The model under review builds one solid part; all positions refer to its coordinate system, in mm. Give positions to 0.01 mm unless a question says otherwise; leave off trailing zeros. Loops run counter-clockwise (first coordinate to the right, second up) from the corner with the lowest first, then second, coordinate; pieces in that order, holes last. Notation, with made-up numbers: (50.5, 50.25) - (84.5, 50.25) arc R31 ccw to (84.5, 76.25) - close; hole circle Ø5 at (33, 48.25). An arc over 180 degrees is marked (long way). Return JSON: item names as keys, results as strings. Group by question number.
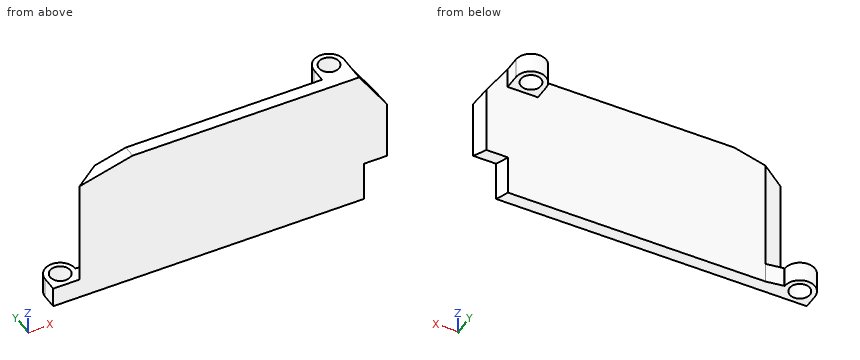
from build123d import *

# Parameters (mm, degrees)
EXTRUDE_1_DEPTH     = 14
CUT_EXTRUDE_1_DEPTH = 4
CUT_EXTRUDE_2_DEPTH = 23.370796565
EXTRUDE_2_DEPTH     = 2
EXTRUDE_3_DEPTH     = 2
MM_1_D              = 2
MM_2_D              = 2


with BuildPart() as part:
    # 草图2 → 凸台-拉伸1 (new body)
    with BuildSketch(Plane(origin=(0, 0, -2), x_dir=(-1, 0, 0), z_dir=(0, 0, -1))):
        with BuildLine():
            Line((-14.855557574, 24.75), (15.584929867, 24.75))
            Line((15.584929867, 24.75), (13.419866357, 26))
            Line((13.419866357, 26), (-14.208438024, 26))
            ThreePointArc((-14.208438024, 26), (-14.507523283, 25.36232965), (-14.855557574, 24.75))
        make_face()
    extrude(amount=EXTRUDE_1_DEPTH)

    # 草图3 → 切除-拉伸1 (cut)
    with BuildSketch(Plane(origin=(0, 0, -16), x_dir=(-1, 0, 0), z_dir=(0, 0, -1))):
        with BuildLine():
            Line((-12.578432584, 24.75), (-17.35825905, 24.75))
            Line((-17.35825905, 24.75), (-16.062803405, 32.25))
            Line((-16.062803405, 32.25), (-11.849295798, 32.25))
            ThreePointArc((-11.849295798, 32.25), (-11.55161702, 28.435617497), (-12.578432584, 24.75))
        make_face()
    extrude(amount=-CUT_EXTRUDE_1_DEPTH, mode=Mode.SUBTRACT)

    # 草图4 → 切除-拉伸2 (cut, through all)
    with BuildSketch(Plane.XZ.offset(-24.75)):
        Polygon((12.09629915, -2), (15.429632483, -7), (15.429632483, -2), align=None)
        Polygon((-10.329335075, -2), (-15.584929867, -3.40823238), (-15.584929867, -2), align=None)
    extrude(amount=-CUT_EXTRUDE_2_DEPTH, mode=Mode.SUBTRACT)

    # 草图6 → 凸台-拉伸2 (add)
    with BuildSketch(Plane(origin=(0, 0, -16), x_dir=(-1, 0, 0), z_dir=(0, 0, -1))):
        with BuildLine():
            Line((13.419866357, 26), (15.584929867, 24.75))
            Line((15.584929867, 24.75), (16.695744446, 24.75))
            ThreePointArc((16.695744446, 24.75), (15.635084274, 25.189339828), (15.195744446, 26.25))
            Line((15.195744446, 26.25), (15.085744446, 26.25))
            Line((15.085744446, 26.25), (13.419866357, 26))
        make_face()
        with BuildLine():
            ThreePointArc((15.195744446, 26.25), (15.635084274, 25.189339828), (16.695744446, 24.75))
            ThreePointArc((16.695744446, 24.75), (17.756404617, 25.189339828), (18.195744446, 26.25))
            Line((18.195744446, 26.25), (15.195744446, 26.25))
        make_face()
        with BuildLine():
            ThreePointArc((18.195744446, 26.25), (16.695744446, 27.75), (15.195744446, 26.25))
            Line((15.195744446, 26.25), (18.195744446, 26.25))
        make_face()
        with BuildLine():
            ThreePointArc((18.195744446, 26.25), (17.756404617, 25.189339828), (16.695744446, 24.75))
            Line((16.695744446, 24.75), (18.195744446, 24.75))
            Line((18.195744446, 24.75), (18.195744446, 26.25))
        make_face()
    extrude(amount=-EXTRUDE_2_DEPTH)

    # 草图7 → 凸台-拉伸3 (add)
    with BuildSketch(Plane.XY.offset(-2)):
        with BuildLine():
            Line((10.59629915, 26), (12.09629915, 26))
            Line((12.09629915, 26), (12.09629915, 27.5))
            ThreePointArc((12.09629915, 27.5), (11.656959321, 26.439339828), (10.59629915, 26))
        make_face()
        with BuildLine():
            Line((9.09629915, 26), (10.59629915, 26))
            ThreePointArc((10.59629915, 26), (9.535638978, 26.439339828), (9.09629915, 27.5))
            Line((9.09629915, 27.5), (9.09629915, 26))
        make_face()
        with BuildLine():
            ThreePointArc((10.59629915, 26), (11.656959321, 26.439339828), (12.09629915, 27.5))
            Line((12.09629915, 27.5), (9.09629915, 27.5))
            ThreePointArc((9.09629915, 27.5), (9.535638978, 26.439339828), (10.59629915, 26))
        make_face()
        with BuildLine():
            Line((9.09629915, 27.5), (12.09629915, 27.5))
            ThreePointArc((12.09629915, 27.5), (10.59629915, 29), (9.09629915, 27.5))
        make_face()
    extrude(amount=-EXTRUDE_3_DEPTH)

    # 大小mm 暗销孔1 (through all)
    with Locations(Plane(origin=(0, 0, -16), x_dir=(-1, 0, 0), z_dir=(0, 0, -1))):
        with Locations((16.691791053, 26.25)):
            Hole(MM_1_D / 2)

    # 大小mm 暗销孔2 (through all)
    with Locations(Plane.XY.offset(-2)):
        with Locations((10.59629915, 27.5)):
            Hole(MM_2_D / 2)


solid = part.part
Item 1: For L1, parallel to Y at x = 4, z = -6.75; L2, parallel to Y at x = -15, z = -9.5; L3, parallel to X at y = 25.75, z = -3.5, list the stretches that pass through material, from the lowest coordinate up. Write a range as from..to.
Item 2: Take a section at A-A (y = 28.05). State the section outline as (x, z) points, then the cut area to 3 significant figures.
Item 3: For P1, Ø1.8, axis at x = 10.6, y = 27.5, coming from the -Z side; P2, Ø3, axis at x = -8, z = -4.5, coming from the +Y side; P3, Ø1.5, axis at x = -15.5, y = 27, coming from the +Z side; P4, Ø1.2, axis at y = 27, z = -3, coming from the -X side, all flat-tipped, find the tip position at first contact; note any pin that passes through.
Item 4: Take a section at C-C (z = -8.5). State the section outline as (x, y) points, then the cut area to 3 significant figures.
Item 5: Take a section at B-B (x = -1.5). State the section outline as (y, z) points, then the cut area to 3 significant figures.
Check sheet entries:
{
 "1": {"L1": "y = 24.75..26", "L2": "y = 24.75..25.09", "L3": "x = -13.85..13.1"},
 "2": {"outline": "(9.2, -4) - (9.76, -4) - (9.76, -2) - (9.2, -2) - close; (11.43, -4) - (11.99, -4) - (11.99, -2) - (11.43, -2) - close", "area": "2.24 mm^2"},
 "3": {"P1": "passes through", "P2": "stops at y = 26", "P3": "stops at z = -14", "P4": "stops at x = 9.1"},
 "4": {"outline": "(-15.58, 24.75) - (14.86, 24.75) arc R9 cw to (14.21, 26) - (-13.42, 26) - close", "area": "36.3 mm^2"},
 "5": {"outline": "(24.75, -16) - (26, -16) - (26, -2) - (24.75, -2) - close", "area": "17.5 mm^2"}
}
